Could you check a few things on this drawing? It's one solid part, dimensions in mm from its lowest x, y, z. Round coordinates to 2 decimals unless told otherwise and drop trailing zeros. Write each loop counter-clockwise with the first axis right and the second up, starting at its lowest first coordinate (ties: lowest second). Pieces come first, ordered by that corner, then holes. Notation, with made-up numbers: (16.25, 46) - (71.25, 46) arc R13 cw to (71.25, 68) - close; hole circle Ø9 at (1, 88.25). An arc over 180 degrees is marked (long way). One line per question, with ' | ' between items. Start each with the question number.
(1) Thinking about a two-plate mould opening in Y: for the marked faces 1, 2, 3 and 4, which applies, pulls with the +Y half, pulls with the -Y half, needs draft (parallel to the pull), parting line crosses it, or undercut?
(2) Imagine slicing it at C-C (x = 1.5). Write out the boundary of the cut face in (y, z), plus the area to 3 significant figures.
(3) Imagine slicing it at B-B (z = 2.5). Write out the boundary of the cut face in (x, y), plus the area to 3 significant figures.
(4) Imagine slicing it at D-D (z = 8). Write out the boundary of the cut face in (x, y), plus the area to 3 significant figures.
(5) Will these pins go through, and if not, where does the flat tip stop? pin 1 (1.6 mm diameter, centred on x = 15, z = 2.5, fed in from -Y); pin 2 (1.5 mm diameter, centred on y = 8, z = 4, fed in from +X); pin 3 (4 mm diameter, centred on x = 6.5, y = 1.5, fed in from -Z).
(6) Imagine slicing it at A-A (x = 5). Write out the boundary of the cut face in (y, z), plus the area to 3 significant figures.
(7) If I drill on L1, parallel to Y at x = 13.75, z = 5; L2, parallel to Z at x = 5, y = 14.85; L3, parallel to Z at x = 15, y = 0.55, over which ranges is the centre line in solid material (lowest first)?
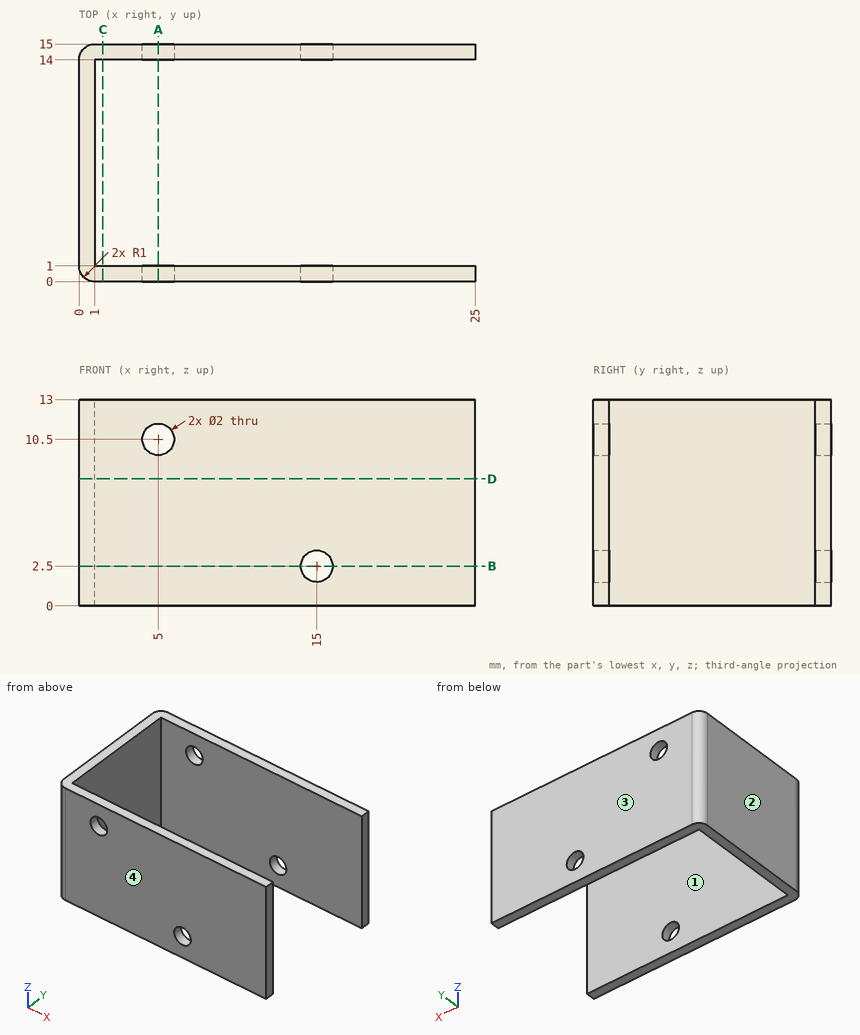
Check sheet entries:
1) face 1: undercut | face 2: needs draft | face 3: pulls with the +Y half | face 4: pulls with the -Y half
2) outline: (0, 0) - (1, 0) - (1, 13) - (0, 13) - close; (14, 0) - (15, 0) - (15, 13) - (14, 13) - close | area: 26.0 mm^2
3) outline: (0, 1) arc R1 ccw to (1, 0) - (14, 0) - (14, 1) - (1, 1) - (1, 14) - (14, 14) - (14, 15) - (1, 15) arc R1 ccw to (0, 14) - close; (16, 0) - (25, 0) - (25, 1) - (16, 1) - close; (16, 14) - (25, 14) - (25, 15) - (16, 15) - close | area: 58.6 mm^2
4) outline: (0, 1) arc R1 ccw to (1, 0) - (25, 0) - (25, 1) - (1, 1) - (1, 14) - (25, 14) - (25, 15) - (1, 15) arc R1 ccw to (0, 14) - close | area: 62.6 mm^2
5) pin 1: through | pin 2: x = 1 | pin 3: z = 0
6) outline: (0, 0) - (1, 0) - (1, 9.5) - (0, 9.5) - close; (0, 11.5) - (1, 11.5) - (1, 13) - (0, 13) - close; (14, 0) - (15, 0) - (15, 9.5) - (14, 9.5) - close; (14, 11.5) - (15, 11.5) - (15, 13) - (14, 13) - close | area: 22.0 mm^2
7) L1: 0 to 1, 14 to 15 | L2: 0 to 9.5, 11.5 to 13 | L3: 0 to 1.5, 3.5 to 13
